Autodesk Inventor part; units mm, degrees
ref_plane "YZ Plane" through (0, 0, 0) normal (1, 0, 0) x (0, 1, 0)
ref_plane "XZ Plane" through (0, 0, 0) normal (0, 1, 0) x (-1, 0, 0)
ref_plane "XY Plane" through (0, 0, 0) normal (0, 0, 1) x (1, 0, 0)
sketch "Sketch1" plane through (0, 0, 0) normal (0, 1, 0) x (-1, 0, 0)
  circle A0 centre (0, 0) radius 25.4
  dimension "d0" = 50.8
extrude "Extrusion1" add sketch "Sketch1" along normal blind 266.7
sketch "Sketch2" plane through (0, 266.7, 0) normal (0, 1, 0) x (1, 0, 0)
  circle A0 centre (0, 0) radius 25.4
  line L0 (-18.3739, -17.5374) -> (18.3739, -17.5374)
  line L1 (18.3739, -17.5374) -> (18.3739, 17.5374)
  line L2 (18.3739, 17.5374) -> (-18.3739, 17.5374)
  line L3 (-18.3739, 17.5374) -> (-18.3739, -17.5374)
  line L4 (-18.3739, -17.5374) -> (18.3739, 17.5374) construction
  line L5 (18.3739, -17.5374) -> (-18.3739, 17.5374) construction
extrude "Extrusion4" add sketch "Sketch2" along normal blind 38.1 contours L1 L0 L3 L2
sketch "Sketch4" plane through (18.3739, 266.7, 17.5374) normal (1, 0, 0) x (0, 0, -1)
  circle A0 centre (17.5374, 19.05) radius 12.7
  point P0 (17.5374, -266.7)
  dimension "d10" = 25.4
extrude "Extrusion5" cut sketch "Sketch4" against normal blind 38.1
sketch "Sketch5" plane through (0, 0, 0) normal (0, -1, 0) x (1, 0, 0)
  circle A0 centre (0, 0) radius 9.525
  dimension "d13" = 19.05
extrude "Extrusion6" cut sketch "Sketch5" against normal blind 266.7
properties part number "cylendar" material "Aluminum 6061"
Can you work these out from the model? Positions are in its coordinate system, mm. A direction names the side the tool comes from. Coordinates: 2 decimals unless noted, no trailing zeros. Loops run counter-clockwise (first coordinate to the right, second up) from the corner with the lowest first, then second, coordinate; pieces in that order, holes last. Notation, with made-up numbers: (-33, 52) - (12, 52) arc R29 cw to (12, 78) - close; hole circle Ø2 at (-16.5, 52). An arc over 180 degrees is marked (long way). Answer as CSV lines item,"result". Start each with the question number.
1) Thinking about a two-plate mould opening in X: for faces 1 (the flat face through (0, 266.7, 0)), 2 (the flat face through (0, 266.7, -21)), 3 (the cylindrical face through (5.506, 131.483, 24.796)), 4 (the flat face through (18.374, 281, 12)), which applies, pulls with the +X half, pulls with the -X half, needs draft (parallel to the pull), parting line crosses it, or undercut?
2) Suppose I cut it at C-C (y = 285.75). Please give me the cut outline in (x, z).
3) I need wall thicknesses on line 1 (Y direction, x = 3, z = 0); line 2 (Z direction, x = 1, y = 83.5); line 3 (Y direction, x = -4.5, z = 19.5). Which ranges of each line are inside material? Lowest first, please. Write a range as from..to.
4) Suppose I cut it at A-A (z = 0). Please give me the cut outline in (x, y) (3 decimals).
5) Which directions (+Z, -Z, +X, -X, +Y, -Y) give clear straight access to the entire face, cutting with the end or side of a thin tool? Please do faces 5 (the flat face through (-21, 266.7, 0)), 6 (the flat face through (0, 266.7, 21)), 7 (the flat face through (0, 285, -17.537)).
6) For pin 1 (2 mm diameter, centred on x = -17.5, y = 160, fed in from -Z); pin 2 (17.5 mm diameter, centred on y = 287.5, z = 3, fed in from -X); pin 3 (10 mm diameter, centred on x = 11, y = 90.5, fed in from -Z); pin 4 (11.5 mm diameter, centred on x = 0, z = 0, fed in from -Y), each with a flat end and sliding along its axis, tell me the tip position at first contact or that it passes through.
7) Suppose I cut it at D-D (y = 166.5). Please give me the cut outline in (x, z) (3 decimals), plus the area to 3 significant figures.
8) Suppose I cut it at B-B (x = 0). Please give me the cut outline in (y, z) (3 decimals).
Check result:
1,face 1,"undercut"
1,face 2,"needs draft"
1,face 3,"parting line crosses it"
1,face 4,"pulls with the +X half"
2,outline,"(-18.37, -17.54) - (18.37, -17.54) - (18.37, -12.7) - (-18.37, -12.7) - close; (-18.37, 12.7) - (18.37, 12.7) - (18.37, 17.54) - (-18.37, 17.54) - close"
3,line 1,"y = 266.7..273.05, 298.45..304.8"
3,line 2,"z = -25.38..-9.47, 9.47..25.38"
3,line 3,"y = 0..266.7"
4,outline,"(-25.4, 0) - (-9.525, 0) - (-9.525, 266.7) - (9.525, 266.7) - (9.525, 0) - (25.4, 0) - (25.4, 266.7) - (18.374, 266.7) - (18.374, 273.05) - (-18.374, 273.05) - (-18.374, 266.7) - (-25.4, 266.7) - close; (-18.374, 298.45) - (18.374, 298.45) - (18.374, 304.8) - (-18.374, 304.8) - close"
5,face 5,"+Z, -Z, -X, +Y"
5,face 6,"+Z, +X, -X, +Y"
5,face 7,"-Z, +X, -X, +Y"
6,pin 1,"stops at z = -19.31"
6,pin 2,"passes through"
6,pin 3,"stops at z = -24.68"
6,pin 4,"stops at y = 266.7"
7,outline,"circle Ø50.8 at (0, 0); hole circle Ø19.05 at (0, 0)"
7,area,"1,740 mm²"
8,outline,"(0, -25.4) - (266.7, -25.4) - (266.7, -17.537) - (304.8, -17.537) - (304.8, 17.537) - (266.7, 17.537) - (266.7, 25.4) - (0, 25.4) - (0, 9.525) - (266.7, 9.525) - (266.7, -9.525) - (0, -9.525) - close; hole circle Ø25.4 at (285.75, 0)"
